from build123d import *

# Parameters (mm, degrees)
BOSS_EXTRUDE1_DEPTH = 12.7
SKETCH2_R           = 3.75
BOSS_EXTRUDE2_DEPTH = 12.7
SKETCH3_R           = 5
BOSS_EXTRUDE3_DEPTH = 2.796


with BuildPart() as part:
    # Sketch1 → Boss-Extrude1 (new body)
    with BuildSketch(Plane.XY):
        Polygon((-7.830526815, 0), (7.830526815, 0), (6.35, 3.175), (-6.35, 3.175), align=None)
    extrude(amount=BOSS_EXTRUDE1_DEPTH)

    # Sketch2 → Boss-Extrude2 (add)
    with BuildSketch(Plane(origin=(0, 3.175, 0), x_dir=(1, 0, 0), z_dir=(0, 1, 0))):
        with Locations(Location((0, -4.708818534, 0), (0, 0, 270))):
            Circle(SKETCH2_R)
    extrude(amount=BOSS_EXTRUDE2_DEPTH)

    # Sketch3 → Boss-Extrude3 (add)
    with BuildSketch(Plane(origin=(0, 3.175, 0), x_dir=(1, 0, 0), z_dir=(0, 1, 0))):
        with Locations(Location((0, -4.708818534, 0), (0, 0, 109.650110836))):
            Circle(SKETCH3_R)
    extrude(amount=BOSS_EXTRUDE3_DEPTH)


solid = part.part
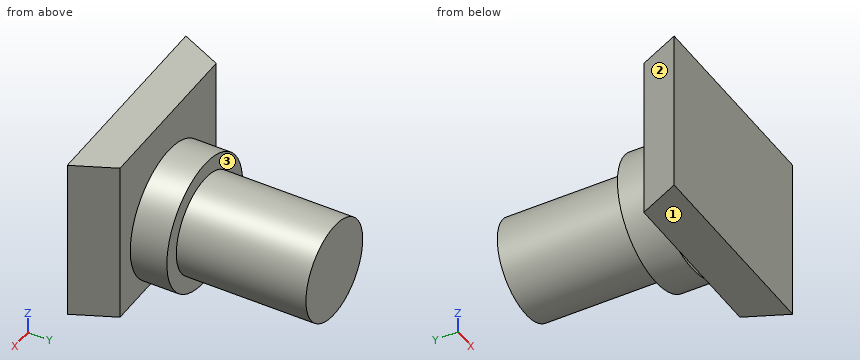
For this review, take the finished solid that the model builds, in its own axes (mm). Face numbers are marked on the shaded views. A direction names the side the tool comes from. Round coordinates to 2 decimals unless told otherwise and drop trailing zeros. Write each loop counter-clockwise with the first axis right and the second up, starting at its lowest first coordinate (ties: lowest second). Pieces come first, ordered by that corner, then holes. Notation, with made-up numbers: (-39.5, -32.5) - (16.5, -32.5) arc R22 cw to (16.5, -23.5) - close; hole circle Ø9 at (9, 50). An arc over 180 degrees is marked (long way). Write item = value, one per line. Start each with the question number.
1. Consider section A-A on x = 0. State the section outline as (y, z) points (3 decimals).
2. For pin 1 Ø5 at (y, z) = (4.5, 8.5) entering from -X; pin 2 Ø2 at (x, y) = (-5, 10) entering from -Z; pin 3 Ø1.6 at (x, y) = (2, 1) entering from -Z; pin 4 Ø6 at (y, z) = (5.5, 6.5) entering from -X, all flat-tipped, find the tip position at first contact; note any pin that passes through.
3. Consider section C-C on y = 5.75. State the section outline as (x, z) points.
4. Wall thickness on L1, parallel to Y at x = 3.5, z = 11.75 (3 decimals); L2, parallel to Z at x = -3.75, y = 2.5; L3, parallel to Y at x = 4.5, z = 6.75: over which ranges is each line inside the solid? List them lowest first.
5. Consider section D-D on x = -4.25. State the section outline as (y, z) points (3 decimals).
6. Consider section B-B on z = 4.75. State the section outline as (x, y) points (3 decimals), plus the area to 3 significant figures.
7. For the marked faces 1, 2 and 3, list the 3-axis set-ups (+Z, -Z, +X, -X, +Y, -Y) from which the entire face can be reached by the end or side of a thin tool; tool diameter is ignored.
Evaluation:
q1.outline = (0, 0) - (3.175, 0) - (3.175, -0.291) - (5.971, -0.291) - (5.971, 0.959) - (15.875, 0.959) - (15.875, 8.459) - (5.971, 8.459) - (5.971, 9.709) - (3.175, 9.709) - (3.175, 12.7) - (0, 12.7) - close
q2.pin_1 = -6.9
q2.pin_2 = through
q2.pin_3 = 0
q2.pin_4 = -6.66
q3.outline = circle Ø10 at (0, 4.71)
q4.L1 = 0 to 3.175
q4.L2 = 0 to 12.7
q4.L3 = 0 to 5.97
q5.outline = (0, 0) - (3.175, 0) - (3.175, 2.075) - (5.971, 2.075) - (5.971, 7.343) - (3.175, 7.343) - (3.175, 12.7) - (0, 12.7) - close
q6.outline = (-7.831, 0) - (7.831, 0) - (6.35, 3.175) - (5, 3.175) - (5, 5.971) - (3.75, 5.971) - (3.75, 15.875) - (-3.75, 15.875) - (-3.75, 5.971) - (-5, 5.971) - (-5, 3.175) - (-6.35, 3.175) - close
q6.area = 147 mm2
q7.face_1 = -Z, +X, -X, -Y
q7.face_2 = +Z, -Z, -X, +Y
q7.face_3 = +Y
